Geometry check sheet. Reference: the model listing, model coordinates, mm. Coordinates: 2 decimals unless noted, no trailing zeros. Write each loop counter-clockwise with the first axis right and the second up, starting at its lowest first coordinate (ties: lowest second). Pieces come first, ordered by that corner, then holes. Notation, with made-up numbers: (-7, -19) -> (43, -19) arc R24 ccw to (43, 8) -> close; hole circle Ø4 at (-4.75, 20). An arc over 180 degrees is marked (long way). Use a Markdown table: item, result.
```python
from build123d import *

# Parameters (mm, degrees)
SKETCH1_W                                         = 46
SKETCH1_H                                         = 15
SKETCH1_R                                         = 4
BOSS_EXTRUDE1_DEPTH                               = 2
CSK_FOR_8_FLAT_HEAD_MACHINE_SCREW_100_D           = 4.9149
CSK_FOR_8_FLAT_HEAD_MACHINE_SCREW_100_DEPTH       = 25
CSK_FOR_8_FLAT_HEAD_MACHINE_SCREW_100_CSINK_D     = 8.4328
CSK_FOR_8_FLAT_HEAD_MACHINE_SCREW_100_CSINK_ANGLE = 100
CSK_FOR_8_FLAT_HEAD_MACHINE_SCREW_100_TIP         = 1.476584928


with BuildPart() as part:
    # Sketch1 → Boss-Extrude1 (new body)
    with BuildSketch(Plane(origin=(0, 0, 0), x_dir=(1, 0, 0), z_dir=(0, 1, 0))):
        Rectangle(SKETCH1_W, SKETCH1_H)
        with Locations(Location((0, 0, 0), (0, 0, 270))):
            Circle(SKETCH1_R, mode=Mode.SUBTRACT)
    extrude(amount=BOSS_EXTRUDE1_DEPTH)

    # CSK for #8 Flat Head Machine Screw (100)1
    with Locations(Plane(origin=(0, 2, 0), x_dir=(1, 0, 0), z_dir=(0, 1, 0))):
        with Locations((-15.5, 0), (15.5, 0)):
            CounterSinkHole(CSK_FOR_8_FLAT_HEAD_MACHINE_SCREW_100_D / 2, CSK_FOR_8_FLAT_HEAD_MACHINE_SCREW_100_CSINK_D / 2, depth=CSK_FOR_8_FLAT_HEAD_MACHINE_SCREW_100_DEPTH, counter_sink_angle=CSK_FOR_8_FLAT_HEAD_MACHINE_SCREW_100_CSINK_ANGLE)
            with Locations((0, 0, -(CSK_FOR_8_FLAT_HEAD_MACHINE_SCREW_100_DEPTH + CSK_FOR_8_FLAT_HEAD_MACHINE_SCREW_100_TIP / 2))):  # 118° drill point
                Cone(0, CSK_FOR_8_FLAT_HEAD_MACHINE_SCREW_100_D / 2, CSK_FOR_8_FLAT_HEAD_MACHINE_SCREW_100_TIP, mode=Mode.SUBTRACT)


solid = part.part
```
Item 1: Section check D-D on z = 2. Count the separate pieces of the cut face and the enclosed holes in it, then the cut area to 3 significant figures.
Answer block:
| item | result |
|---|---|
| separate pieces | 4 |
| enclosed holes | 0 |
| area | 59.6 mm^2 |
Item 2: Section check B-B on x = 15.5. Record the boundary of the cut face in (y, z).
Answer block:
| item | result |
|---|---|
| outline | (0, -7.5) -> (2, -7.5) -> (2, -4.22) -> (0.52, -2.46) -> (0, -2.46) -> close; (0, 2.46) -> (0.52, 2.46) -> (2, 4.22) -> (2, 7.5) -> (0, 7.5) -> close |
Item 3: Section check C-C on x = 0.5. Record the boundary of the cut face in (y, z), then the cut area to 3 significant figures.
Answer block:
| item | result |
|---|---|
| outline | (0, -7.5) -> (2, -7.5) -> (2, -3.97) -> (0, -3.97) -> close; (0, 3.97) -> (2, 3.97) -> (2, 7.5) -> (0, 7.5) -> close |
| area | 14.1 mm^2 |
Item 4: Section check A-A on z = 0. Record the boundary of the cut face in (x, y), then the cut area to 3 significant figures.
Answer block:
| item | result |
|---|---|
| outline | (-23, 0) -> (-17.96, 0) -> (-17.96, 0.52) -> (-19.72, 2) -> (-23, 2) -> close; (-13.04, 0) -> (-4, 0) -> (-4, 2) -> (-11.28, 2) -> (-13.04, 0.52) -> close; (4, 0) -> (13.04, 0) -> (13.04, 0.52) -> (11.28, 2) -> (4, 2) -> close; (17.96, 0) -> (23, 0) -> (23, 2) -> (19.72, 2) -> (17.96, 0.52) -> close |
| area | 51.1 mm^2 |
Item 5: Mould release check, pull along X, two halves, no side actions. Record for faces 1 (the flat face through (-23, 1, 0)), 2 (the cylindrical face through (-17.844, 0.258, -0.738)), 3 (the flat face through (0, 0, 5)): +X half, -X half, draft (parallel to the pull), parting line (faces both ways), or undercut.
Answer block:
| item | result |
|---|---|
| face 1 | -X half |
| face 2 | undercut |
| face 3 | draft |
Item 6: Thickness scan on L1, parallel to Z at x = -15.5, y = 0.45; L2, parallel to Z at x = -14.5, y = 0.9; L3, parallel to X at y = 0.8, z = 3.25. Record the ranges inside material, lowest first. Write a range as [from, to].
Answer block:
| item | result |
|---|---|
| L1 | z = [-7.5, -2.46], [2.46, 7.5] |
| L2 | z = [-7.5, -2.73], [2.73, 7.5] |
| L3 | x = [-23, -2.33], [2.33, 23] |
Item 7: Depth check by flat-ended pin: P1, Ø6.5, axis at x = 15.5, z = 0, coming from the +Y side. Enter the tip coordinate at first touch or a pass-through.
Answer block:
| item | result |
|---|---|
| P1 | stops at y = 1.19 |
